from build123d import *

# Parameters (mm, degrees)
F1_DEPTH = 10.16


with BuildPart() as f1:
    # F0 (on Top) → F1 (new body)
    with BuildSketch(Plane.XY):
        with BuildLine():
            ThreePointArc((9.556043, 26.255012), (6.934197, 33.917019), (0, 38.1))
            Line((0, 38.1), (0, 27.94))
            ThreePointArc((0, 27.94), (-5.08429, 34.243207), (-13.030967, 35.802289))
            Line((-13.030967, 35.802289), (-9.556043, 26.255012))
            ThreePointArc((-9.556043, 26.255012), (-16.489536, 30.43916), (-24.490208, 29.186293))
            Line((-24.490208, 29.186293), (-17.959486, 21.403282))
            ThreePointArc((-17.959486, 21.403282), (-25.905901, 22.9637), (-32.995568, 19.05))
            Line((-32.995568, 19.05), (-24.19675, 13.97))
            ThreePointArc((-24.19675, 13.97), (-32.197632, 12.71848), (-37.521175, 6.615996))
            Line((-37.521175, 6.615996), (-27.515529, 4.85173))
            ThreePointArc((-27.515529, 4.85173), (-34.605854, 0.939223), (-37.521175, -6.615996))
            Line((-37.521175, -6.615996), (-27.515529, -4.85173))
            ThreePointArc((-27.515529, -4.85173), (-32.840098, -10.953318), (-32.995568, -19.05))
            Line((-32.995568, -19.05), (-24.19675, -13.97))
            ThreePointArc((-24.19675, -13.97), (-27.113343, -21.524728), (-24.490208, -29.186293))
            Line((-24.490208, -29.186293), (-17.959486, -21.403282))
            ThreePointArc((-17.959486, -21.403282), (-18.116318, -29.499937), (-13.030967, -35.802289))
            Line((-13.030967, -35.802289), (-9.556043, -26.255012))
            ThreePointArc((-9.556043, -26.255012), (-6.934197, -33.917019), (0, -38.1))
            Line((0, -38.1), (0, -27.94))
            ThreePointArc((0, -27.94), (5.08429, -34.243207), (13.030967, -35.802289))
            Line((13.030967, -35.802289), (9.556043, -26.255012))
            ThreePointArc((9.556043, -26.255012), (16.489536, -30.43916), (24.490208, -29.186293))
            Line((24.490208, -29.186293), (17.959486, -21.403282))
            ThreePointArc((17.959486, -21.403282), (25.905901, -22.9637), (32.995568, -19.05))
            Line((32.995568, -19.05), (24.19675, -13.97))
            ThreePointArc((24.19675, -13.97), (32.197632, -12.71848), (37.521175, -6.615996))
            Line((37.521175, -6.615996), (27.515529, -4.85173))
            ThreePointArc((27.515529, -4.85173), (34.605854, -0.939223), (37.521175, 6.615996))
            Line((37.521175, 6.615996), (27.515529, 4.85173))
            ThreePointArc((27.515529, 4.85173), (32.840098, 10.953318), (32.995568, 19.05))
            Line((32.995568, 19.05), (24.19675, 13.97))
            ThreePointArc((24.19675, 13.97), (27.113343, 21.524728), (24.490208, 29.186293))
            Line((24.490208, 29.186293), (17.959486, 21.403282))
            ThreePointArc((17.959486, 21.403282), (18.116318, 29.499937), (13.030967, 35.802289))
            Line((13.030967, 35.802289), (9.556043, 26.255012))
        make_face()
    extrude(amount=F1_DEPTH)


solid = f1.part
Could you check a few things on this model? Use its own coordinates, in mm. Give positions to 0.01 mm unless a question says otherwise; leave off trailing zeros. Order: outer loops, then holes, each group sorted by start corner. A loop starts at its lowest first (then second) coordinate and runs counter-clockwise, first axis right, second up.
1. I need wall thicknesses on L1, parallel to X at y = -22, z = 7.5; L2, parallel to X at y = -29, z = 7; L3, parallel to Y at x = -25.5, z = 8. Which ranges of each line are inside material? Lowest first, please.
2. Suppose I cut it at A-A (x = 21.5). List the corners of the cut face in (y, z) for me, plus the area to 3 significant figures.
3. Suppose I cut it at C-C (y = -10.5). List the corners of the cut face in (x, z) for me.
4. Will these pins go through, and if not, where does the flat tip stop? P1, Ø3, axis at x = 15.5, z = 6.5, coming from the -Y side; P2, Ø5, axis at y = -2.5, z = 5, coming from the +X side; P3, Ø5, axis at y = -31, z = 4.5, coming from the +X side.
5. Suppose I cut it at B-B (x = -8). List the corners of the cut face in (y, z) for me.
Solved:
1. L1: x = -27.11 to -18.46, -18.17 to 18.46, 19.08 to 29.07
1. L2: x = -24.64 to -24.33, -18.28 to -10.56, -9.29 to 0, 0.42 to 10.56, 12.72 to 24.33
1. L3: y = -27.72 to -15.78, -14.72 to 14.15, 14.72 to 23.02
2. outline: (-30.34, 0) - (-25.62, 0) - (-25.62, 10.16) - (-30.34, 10.16) - close; (-22.82, 0) - (25.62, 0) - (25.62, 10.16) - (-22.82, 10.16) - close
2. area: 540 mm2
3. outline: (-32.65, 0) - (35.07, 0) - (35.07, 10.16) - (-32.65, 10.16) - close
4. P1: stops at y = -30.53
4. P2: stops at x = 35.35
4. P3: stops at x = 24.49
5. outline: (-32.36, 0) - (35.5, 0) - (35.5, 10.16) - (-32.36, 10.16) - close
